Geometry check sheet. Reference: the model listing, model coordinates, mm. A direction names the side the tool comes from. Round coordinates to 2 decimals unless told otherwise and drop trailing zeros. Write each loop counter-clockwise with the first axis right and the second up, starting at its lowest first coordinate (ties: lowest second). Pieces come first, ordered by that corner, then holes. Notation, with made-up numbers: (60.5, 77.25) - (77.5, 77.25) arc R14 ccw to (77.5, 81.25) - close; hole circle Ø2 at (-30.5, 56.25). An arc over 180 degrees is marked (long way). Return JSON: item names as keys, results as strings. Group by question number.
from build123d import *

# Parameters (mm, degrees)
F0_R     = 3
F0_R_2   = 1.5
F1_DEPTH = 20


with BuildPart() as f1:
    # F0 (on Top) → F1 (new body)
    with BuildSketch(Plane.XY):
        Circle(F0_R)
        Circle(F0_R_2, mode=Mode.SUBTRACT)
        with Locations((-10, 0)):
            Circle(F0_R)
        with Locations((-10, 0)):
            Circle(F0_R_2, mode=Mode.SUBTRACT)
        with Locations((-10, -10)):
            Circle(F0_R)
        with Locations((-10, -10)):
            Circle(F0_R_2, mode=Mode.SUBTRACT)
        with Locations((0, -10)):
            Circle(F0_R)
        with Locations((0, -10)):
            Circle(F0_R_2, mode=Mode.SUBTRACT)
    extrude(amount=F1_DEPTH)

    # F2 (on Right) → F3 (revolve)
    with BuildSketch(Plane.YZ):
        Polygon((0, 3.5), (0, 0), (5.1, 0), (3, 3.5), align=None)
    revolve(axis=Axis((0, 0, 1.75), (0, 0, 1)))

    # F2 (on Right) → F4 (revolve)
    with BuildSketch(Plane.YZ):
        Polygon((-15.1, 0), (-10, 0), (-10, 3.5), (-13, 3.5), align=None)
    revolve(axis=Axis((0, -10, 1.75), (0, 0, 1)))

    # F6 (on offset) → F7 (revolve)
    with BuildSketch(Plane.YZ.offset(-10)):
        Polygon((0, 3.5), (0, 0), (5.1, 0), (3, 3.5), align=None)
    revolve(axis=Axis((-10, 0, 1.75), (0, 0, 1)))

    # F6 (on offset) → F8 (revolve)
    with BuildSketch(Plane.YZ.offset(-10)):
        Polygon((-15.1, 0), (-10, 0), (-10, 3.5), (-13, 3.5), align=None)
    revolve(axis=Axis((-10, -10, 1.75), (0, 0, 1)))


solid = f1.part
1. Mould release check, pull along Y, two halves, no side actions. Record for faces 1 (the face through (-0.93, 2.96, 3.33)), 2 (the face through (-8.7, -1.3, 20)): pulls with the +Y half, pulls with the -Y half, needs draft (parallel to the pull), parting line crosses it, or undercut.
2. Section check B-B (x = 0). Enter the section's corners in (y, z).
3. Material ranges on line 1 along Y through (x, z) = (-10, 14.75); line 2 along Y through (x, z) = (-11.25, 15.5), recorded low to high.
4. Depth check by flat-ended pin: pin 1 Ø12 at (y, z) = (-4.5, 13.5) entering from -X; pin 2 Ø1.5 at (x, y) = (0.5, -0.5) entering from +Z; pin 3 Ø6 at (y, z) = (-3.5, 5) entering from +X; pin 4 Ø1 at (y, z) = (-6, 16) entering from +X. Enter the tip coordinate at first touch or a pass-through.
5. Section check A-A (z = 15.5). Enter the section's corners in (x, y), and give its area (3 significant figures).
6. Tool access check on faces 3 (the face through (-7.14, -9.1, 11.63)), 4 (the face through (-8.7, -11.3, 20)). Record the directions out of +Z, -Z, +X, -X, +Y, -Y that give a thin tool (end or side, any length) a straight path to the whole face; none if there is none.
Result sheet:
{
 "1": {"face 1": "undercut", "face 2": "needs draft"},
 "2": {"outline": "(-15.1, 0) - (5.1, 0) - (3, 3.5) - (3, 20) - (1.5, 20) - (1.5, 3.5) - (-1.5, 3.5) - (-1.5, 20) - (-3, 20) - (-3, 3.5) - (-5, 0.17) - (-7, 3.5) - (-7, 20) - (-8.5, 20) - (-8.5, 3.5) - (-11.5, 3.5) - (-11.5, 20) - (-13, 20) - (-13, 3.5) - close"},
 "3": {"line 1": "y = -13 to -11.5, -8.5 to -7, -3 to -1.5, 1.5 to 3", "line 2": "y = -12.73 to -10.83, -9.17 to -7.27, -2.73 to -0.83, 0.83 to 2.73"},
 "4": {"pin 1": "stops at x = -13", "pin 2": "stops at z = 3.5", "pin 3": "stops at x = 3.11", "pin 4": "passes through"},
 "5": {"outline": "circle Ø6 at (-10, -10); circle Ø6 at (-10, 0); circle Ø6 at (0, -10); circle Ø6 at (0, 0); hole circle Ø3 at (-10, -10); hole circle Ø3 at (-10, 0); hole circle Ø3 at (0, -10); hole circle Ø3 at (0, 0)", "area": "84.8 mm²"},
 "6": {"face 3": "+Z", "face 4": "+Z, +X, -X, +Y, -Y"}
}
